```python
from build123d import *

# Parameters (mm, degrees)
SKETCH1_R           = 1.6
BOSS_EXTRUDE1_DEPTH = 7.5
SKETCH2_R           = 5.075
SKETCH2_R_2         = 1.6
CUT_EXTRUDE1_DEPTH  = 3.75
FILLET1_R           = 5
SKETCH3_R           = 5
CUT_EXTRUDE2_DEPTH  = 3.9
CUT_EXTRUDE5_DEPTH  = 8.5
FILLET2_R           = 1
FILLET3_R           = 1


with BuildPart() as part:
    # Sketch1 → Boss-Extrude1 (new body)
    with BuildSketch(Plane.XY):
        with BuildLine():
            Line((10, 5), (10, 7.5))
            Line((10, 7.5), (-10, 7.5))
            Line((-10, 7.5), (-10, -7.5))
            Line((-10, -7.5), (10, -7.5))
            Line((10, -7.5), (10, -5))
            ThreePointArc((10, -5), (15, 0), (10, 5))
        make_face()
        with Locations((10, 0)):
            Circle(SKETCH1_R, mode=Mode.SUBTRACT)
    extrude(amount=BOSS_EXTRUDE1_DEPTH)

    # Sketch2 → Cut-Extrude1 (cut)
    with BuildSketch(Plane.XY.offset(7.5)):
        with Locations((-10, 0)):
            Circle(SKETCH2_R)
        with Locations((-10, 0)):
            Circle(SKETCH2_R_2, mode=Mode.SUBTRACT)
    extrude(amount=-CUT_EXTRUDE1_DEPTH, mode=Mode.SUBTRACT)

    # Fillet1
    fillet1_edges = [part.edges().sort_by_distance(p)[0] for p in [
        (0, -7.5, 0),
        (0, 7.5, 0),
    ]]
    fillet(fillet1_edges, radius=FILLET1_R)

    # Sketch3 → Cut-Extrude2 (cut)
    with BuildSketch(Plane(origin=(0, 0, 0), x_dir=(-1, 0, 0), z_dir=(0, 0, -1))):
        with Locations((-10, 0)):
            Circle(SKETCH3_R)
    extrude(amount=-CUT_EXTRUDE2_DEPTH, mode=Mode.SUBTRACT)

    # Sketch5 → Cut-Extrude5 (cut, through all)
    with BuildSketch(Plane(origin=(0, 0, 0), x_dir=(-1, 0, 0), z_dir=(0, 0, -1))):
        with BuildLine():
            Line((-6.464466094, -3.535533906), (-2.5, -7.5))
            Line((-2.5, -7.5), (-10, -7.5))
            Line((-10, -7.5), (-10, -5))
            ThreePointArc((-10, -5), (-8.086582838, -4.619397663), (-6.464466094, -3.535533906))
        make_face()
    extrude(amount=-CUT_EXTRUDE5_DEPTH, mode=Mode.SUBTRACT)

    # Fillet2
    fillet2_edges = [part.edges().sort_by_distance(p)[0] for p in [
        (6.464466094, -3.535533906, 2.00420414),
    ]]
    fillet(fillet2_edges, radius=FILLET2_R)

    # Mirror2: part across plane


with BuildPart() as part_1:
    add(part.part)
    add(part.part.mirror(Plane(origin=(10, 0, 7.5), x_dir=(1, 0, 0), z_dir=(0, 0, 1))))

    # Fillet3
    fillet3_edges = [part_1.edges().sort_by_distance(p)[0] for p in [
        (6.464466094, -3.535533906, 7.5),
    ]]
    fillet(fillet3_edges, radius=FILLET3_R)


solid = part_1.part
```
Geometry: final body of the model. Coordinates: model frame, mm. A direction names the side the tool comes from. Round coordinates to 2 decimals unless told otherwise and drop trailing zeros. Loops run counter-clockwise (first coordinate to the right, second up) from the corner with the lowest first, then second, coordinate; pieces in that order, holes last.
Item 1: Mould query, pull axis Y, two halves, no side actions, for faces 5 (the cylindrical face through (14.72, -1.65, 7.55)), 6 (the cylindrical face through (6.1, -3.6, 13)), 7 (the flat face through (-10, 0, 8)). Classes: released by +Y, released by -Y, zero draft, split by the parting line, or undercut.
Checked values:
face 5: split by the parting line
face 6: undercut
face 7: zero draft
Item 2: Line query: L1, parallel to X at y = 0, z = 6.5 (3 decimals); L2, parallel to Z at x = -7.5, y = -2.25; L3, parallel to X at y = -1.25, z = 8. Output: solid intervals per line, ascending.
Checked values:
L1: x = -10 to -8.4, -4.925 to 8.4, 11.6 to 15
L2: z = 0 to 3.75, 11.25 to 15
L3: x = -10 to -9, -5.08 to 9, 11 to 14.84
Item 3: Section B-B, the plane z = 10.5. Output: boundary loops of the cut face in (x, y) (3 decimals).
Checked values:
outline: (-10, -7.475) - (2.525, -7.475) - (5.817, -4.183) arc R1 cw to (7.103, -4.075) arc R5 ccw (long way) to (10, 5) - (10, 7.475) - (-10, 7.475) - (-10, 5.075) arc R5.075 cw to (-10, -5.075) - close; (-10, -1.6) arc R1.6 ccw to (-10, 1.6) - close; hole circle Ø3.2 at (10, 0)
Item 4: Section A-A, the plane y = 0. Output: boundary loops of the cut face in (x, z) (3 decimals), plus the area to 3 significant figures.
Checked values:
outline: (-10, 0) - (5, 0) - (5, 3.9) - (8.4, 3.9) - (8.4, 11.1) - (5, 11.1) - (5, 15) - (-10, 15) - close; (11.6, 3.9) - (15, 3.9) - (15, 11.1) - (11.6, 11.1) - close; hole (-8.4, 3.75) - (-4.925, 3.75) - (-4.925, 11.25) - (-8.4, 11.25) - close
area: 248 mm2
Item 5: Section D-D, the plane z = 5.75. Output: boundary loops of the cut face in (x, y) (3 decimals).
Checked values:
outline: (-10, -7.5) - (2.5, -7.5) - (5.817, -4.183) arc R1 cw to (7.103, -4.075) arc R5 ccw (long way) to (10, 5) - (10, 7.5) - (-10, 7.5) - (-10, 5.075) arc R5.075 cw to (-10, -5.075) - close; (-10, -1.6) arc R1.6 ccw to (-10, 1.6) - close; hole circle Ø3.2 at (10, 0)
Item 6: Section C-C, the plane x = 11.25. Output: boundary loops of the cut face in (y, z).
Checked values:
outline: (-4.84, 3.9) - (-1, 3.9) - (-1, 11.1) - (-4.84, 11.1) - close; (1, 3.9) - (4.84, 3.9) - (4.84, 11.1) - (1, 11.1) - close
Item 7: Contact query for flat-ended pins moving along their axis: P1, Ø1, axis at x = 5.5, z = 5, coming from the -Y side; P2, Ø2, axis at y = 6.5, z = 8.5, coming from the +X side; P3, Ø1.5, axis at y = 3.5, z = 3.5, coming from the +X side; P4, Ø1.9, axis at x = 10, y = 0, coming from the +Z side. Output: stop coordinate, or through.
Checked values:
P1: stops at y = -5
P2: stops at x = 10
P3: stops at x = 14.1
P4: passes through
Item 8: Reachability of faces 1 (the flat face through (-7, 0, 3.75)), 2 (the cylindrical face through (5.52, 2.22, 13.08)), 3 (the cylindrical face through (6.1, -3.6, 2)), 4 (the flat face through (4, -6, 8)) from +Z, -Z, +X, -X, +Y, -Y: full face, straight path, thin tool, end or side. Return the list, or none.
Checked values:
face 1: none
face 2: +Z, +X
face 3: -Z, +X
face 4: +Z, -Z, -Y
